For this review, take the finished solid that the model builds, in its own axes (mm). A direction names the side the tool comes from. Round coordinates to 2 decimals unless told otherwise and drop trailing zeros. Write each loop counter-clockwise with the first axis right and the second up, starting at its lowest first coordinate (ties: lowest second). Pieces come first, ordered by that corner, then holes. Notation, with made-up numbers: M -19,-10.75 L 9,-10.75 A33 cw 9,18.25 Z; hole C -10,6.5 d1. An arc over 180 degrees is marked long. One line per question, with ' | ' between items.
```python
from build123d import *

# Parameters (mm, degrees)
F0_W      = 45
F0_H      = 25
F1_DEPTH  = 1380
F3_DEPTH  = 45
F5_DEPTH  = 45
F6_W      = 45
F6_H      = 18.5474166647
F7_DEPTH  = 1380
F9_DEPTH  = 45
F11_DEPTH = 45


with BuildPart() as f1:
    # F0 (on Front) → F1 (new body)
    with BuildSketch(Plane.XZ):
        Rectangle(F0_W, F0_H)
    extrude(amount=-F1_DEPTH)

    # F2 (on face) → F3 (cut)
    with BuildSketch(Plane.YZ.offset(22.5)):
        Polygon((0, 12.5), (0, -12.5), (25, 12.5), align=None)
    extrude(amount=-F3_DEPTH, mode=Mode.SUBTRACT)

    # F4 (on face) → F5 (cut)
    with BuildSketch(Plane(origin=(-22.5, 0, 0), x_dir=(0, -1, 0), z_dir=(-1, 0, 0))):
        Polygon((-1380, 12.5), (-1380, -12.5), (-1355, 12.5), align=None)
    extrude(amount=-F5_DEPTH, mode=Mode.SUBTRACT)

    # F6 (on Front) → F7 (join)
    with BuildSketch(Plane.XZ):
        with Locations((0, 21.7737083323)):
            Rectangle(F6_W, F6_H)
    extrude(amount=-F7_DEPTH)

    # F8 (on face) → F9 (cut)
    with BuildSketch(Plane.YZ.offset(22.5)):
        Polygon((70, 31.0474166647), (0, 31.0474166647), (0, 12.5), (25, 12.5), (70, 12.5), align=None)
    extrude(amount=-F9_DEPTH, mode=Mode.SUBTRACT)

    # F10 (on face) → F11 (cut)
    with BuildSketch(Plane.YZ.offset(22.5)):
        Polygon((1355, 12.5), (1380, 12.5), (1380, 31.0474166647), (1310, 31.0474166647), (1310, 12.5), align=None)
    extrude(amount=-F11_DEPTH, mode=Mode.SUBTRACT)


solid = f1.part
```
Item 1: Machinability: for faces 1 (the face through (0, 1332, 12.5)), 2 (the face through (0, 47, 12.5)), 3 (the face through (0, 680, -12.5)), which of the approach directions +Z, -Z, +X, -X, +Y, -Y give a long, thin tool a straight path to every point of the face, cutting with its end or side? Answer none if there is none.
Results:
face 1: +Z, +X, -X, +Y | face 2: +Z, +X, -X, -Y | face 3: -Z, +X, -X, +Y, -Y
Item 2: Insertion check: pin 1 Ø9.5 at (x, z) = (9.5, 24.5) entering from +Y; pin 2 Ø3 at (x, z) = (-2, -5.5) entering from -Y; pin 3 Ø3 at (x, z) = (9, 10.5) entering from +Y. Each pin has a flat end and moves straight along its axis. Give the tip position at first contact, or say it passes through.
Results:
pin 1: y = 1310 | pin 2: y = 5.5 | pin 3: y = 1358.5
Item 3: To check wall thickness, follow line 1 along Y through (x, z) = (-13, 28.5); line 2 along Y through (x, z) = (-18, 9.5). State the ranges of each line that lie inside material, in increasing order. Write a range as from..to.
Results:
line 1: 70..1310 | line 2: 22..1358
Item 4: Take a section at A-A (x = 8). Write out the cut boundary in (y, z), then the cut area to 3 significant figures.
Results:
outline: M 0,-12.5 L 1380,-12.5 L 1355,12.5 L 1310,12.5 L 1310,31.05 L 70,31.05 L 70,12.5 L 25,12.5 Z | area: 56,900 mm2
